Autodesk Fusion 360 part; units mm, degrees
sketch "Sketch1" plane through (0, 0, 0) normal (0, 1, 0) x (1, 0, 0)
  line L0 (0, 0) -> (50, 0) construction
  circle A0 centre (50, 0) radius 10
  circle A1 centre (0, 0) radius 10
  arc A2 (42.8571, -18.681) -> (7.1429, -18.681) centre (25, -65.3835) ccw
  arc A3 (7.1429, 18.681) -> (42.8571, 18.681) centre (25, 65.3835) ccw
  arc A4 (7.1429, 18.681) -> (7.1429, -18.681) centre (0, 0) ccw
  arc A5 (42.8571, -18.681) -> (42.8571, 18.681) centre (50, 0) ccw
  dimension "d13" = 50
  dimension "d14" = 40
  dimension "d15" = 40
  dimension "d16" = 20
  dimension "d17" = 20
  dimension "d18" = 100
  dimension "d19" = 100
extrude "Extrude1" add sketch "Sketch1" along normal blind 3
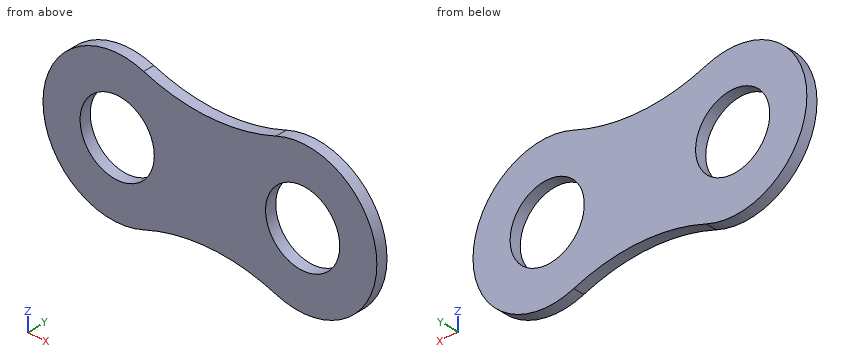
Here's how the part is built. I have some questions about the finished solid (model axes, mm). Coordinates: 2 decimals unless noted, no trailing zeros. Order: outer loops, then holes, each group sorted by start corner. A loop starts at its lowest first (then second) coordinate and runs counter-clockwise, first axis right, second up.
Item 1: For P1, Ø1.5, axis at y = 1, z = 12, coming from the -X side; P2, Ø1.5, axis at x = 59, y = 1.5, coming from the +Z side; P3, Ø1, axis at x = 2.5, y = 2.5, coming from the +Z side, each with a flat end and sliding along its axis, tell me the tip position at first contact or that it passes through.
Result sheet:
P1: stops at x = -16.54
P2: stops at z = 18.22
P3: stops at z = 19.9
Item 2: If we section it at B-B on z = 0: List the corners of the cut face in (x, y) for me, plus the area to 3 significant figures.
Result sheet:
outline: (-20, 0) - (-10, 0) - (-10, 3) - (-20, 3) - close; (10, 0) - (40, 0) - (40, 3) - (10, 3) - close; (60, 0) - (70, 0) - (70, 3) - (60, 3) - close
area: 150 mm2
Item 3: If we section it at C-C on y = 0.6: List the corners of the cut face in (x, z) for me.
Result sheet:
outline: (7.14, -18.68) arc R50 cw to (42.86, -18.68) arc R20 ccw (long way) to (42.86, 18.68) arc R50 cw to (7.14, 18.68) arc R20 ccw (long way) to start; hole circle Ø20 at (0, 0); hole circle Ø20 at (50, 0)
Item 4: If we section it at A-A on x = 50: List the corners of the cut face in (y, z) for me, plus the area to 3 significant figures.
Result sheet:
outline: (0, -20) - (3, -20) - (3, -10) - (0, -10) - close; (0, 10) - (3, 10) - (3, 20) - (0, 20) - close
area: 60.0 mm2
Item 5: I need wall thicknesses on line 1 (X direction, y = 2.95, z = 2); line 2 (Z direction, x = 0, y = 2.3); line 3 (X direction, y = 1.4, z = -5). Which ranges of each line are inside material? Lowest first, please.
Result sheet:
line 1: x = -19.9 to -9.8, 9.8 to 40.2, 59.8 to 69.9
line 2: z = -20 to -10, 10 to 20
line 3: x = -19.36 to -8.66, 8.66 to 41.34, 58.66 to 69.36
Item 6: If we section it at D-D on z = 17: List the corners of the cut face in (x, y) for me, plus the area to 3 significant figures.
Result sheet:
outline: (-10.54, 0) - (12.39, 0) - (12.39, 3) - (-10.54, 3) - close; (37.61, 0) - (60.54, 0) - (60.54, 3) - (37.61, 3) - close
area: 138 mm2
